from build123d import *

# Parameters (mm, degrees)
F0_R     = 11.5
F1_DEPTH = 2
F2_R     = 11.5
F2_R_2   = 9.5
F3_DEPTH = 0.4
F4_R     = 1.25
F5_DEPTH = 0.4
F6_R     = 0.39999


# Not quite as in the source:
# - a fillet or chamfer is up to 0.001 mm smaller than in the source, because OpenCascade refuses the exact size


with BuildPart() as f1:
    # F0 (on Top) → F1 (new body)
    with BuildSketch(Plane.XY):
        Circle(F0_R)
    extrude(amount=F1_DEPTH)

    # F2 (on face) → F3 (join)
    with BuildSketch(Plane.XY.offset(2)):
        Circle(F2_R)
        Circle(F2_R_2, mode=Mode.SUBTRACT)
    extrude(amount=F3_DEPTH)

    # F4 (on face) → F5 (join)
    with BuildSketch(Plane.XY.offset(2)):
        Polygon((-4.9462847407, 4.6223603384), (-6.7446869929, 4.6223603384), (-6.7446869929, 3.631329312), (-5.5307656769, 3.631329312), (-3.7330235863, -2.611553217), (4.2630984261, -2.611553217), (4.2630984261, -1.7084874132), (-2.6016419292, -1.7084874132), (5.1088749777, -0.4323172916), (5.1088749777, 3.1326496529), (-4.5172977159, 3.1326496529), align=None)
        Polygon((-3.1724679652, -0.8662961763), (-4.0021237171, 2.0147863915), (3.9558067254, 2.0147863915), (3.9558067254, 0.3135068497), align=None, mode=Mode.SUBTRACT)
        with Locations((-2.7432420498, -4.2344009733)):
            Circle(F4_R)
        with Locations((3.0116447943, -4.2793590558)):
            Circle(F4_R)
    extrude(amount=F5_DEPTH)

    # F6 (radius 0.4 in the source; OpenCascade refuses exactly that, so slightly less here)
    f6_edges = [f1.edges().sort_by_distance(p)[0] for p in [
        (-11.5, 0, 2.4),
        (-9.5, 0, 2.4),
        (-11.5, 0, 0),
    ]]
    fillet(f6_edges, radius=F6_R)


solid = f1.part
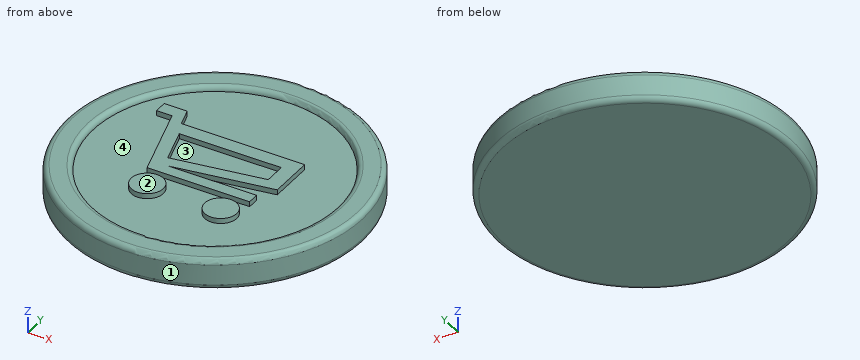
Model file for the job. Use its own axes, mm. Face numbers are marked on the shaded views. Give positions to 0.01 mm unless a question says otherwise; leave off trailing zeros. Order: outer loops, then holes, each group sorted by start corner. A loop starts at its lowest first (then second) coordinate and runs counter-clockwise, first axis right, second up. Notation, with made-up numbers: M 84,-39 L 140,-39 A29 cw 140,-7 Z; hole C 43.5,-12 d11. An arc over 180 degrees is marked long. Write item = value, one per line.
Q1. Flat gauge pins, fed straight in: pin 1 (1 mm diameter, centred on x = -7, y = -1, fed in from +Z); pin 2 (1 mm diameter, centred on x = 9, z = 1.5, fed in from -Y). Where does each tip first touch, or does it go through?
Derived:
pin_1 = 2
pin_2 = -7.75
Q2. Drill centre lines: line 1 (Y direction, x = 0, z = 2.05); line 2 (Z direction, x = -6.5, y = 3); line 3 (Y direction, x = 6.75, z = 2.1). Where is each one in solid material? Low to high. Write a range as [from, to].
Derived:
line_1 = [-11.5, -9.5], [-2.61, -1.71], [-1.28, -0.34], [2.01, 3.13], [9.5, 11.5]
line_2 = [0, 2]
line_3 = [-9.29, -6.7], [6.7, 9.29]
Q3. Two-plate mould, pull along X, no slides. Class the marked faces 1, 2, 3 and 4: pulls with the +X half, pulls with the -X half, needs draft (parallel to the pull), parting line crosses it, or undercut.
Derived:
face_1 = parting line crosses it
face_2 = needs draft
face_3 = undercut
face_4 = undercut
Q4. Cut at C-C, the plane z = 1.5. List the corners of the cut face in (x, y).
Derived:
outline = C 0,0 d23
